from build123d import *

# Parameters (mm, degrees)
HEXBASE_DEPTH             = 2
TUBECLAMPINGHEADS_R       = 5.9
TUBECLAMPINGHEAD_DEPTH    = 2
FASTENINGHEADS_R          = 6.5785
FASTENINGHEAD_DEPTH       = 8
FASTENINGHEAD_TAPER       = 2.5
BOREFASTENINGHEADS_R      = 4.7
BOREFASTENINGHEAD_DEPTH   = 3.2
HEXKEY_DEPTH              = 16.197806859
BORETUBEACCESSS_R         = 5
BORETUBEACCESS_DEPTH      = 9.8
ORINGSEAT_START           = 1.5
ORINGSEATS_R              = 5
ORINGSEATS_R_2            = 4
ORINGSEAT_DEPTH           = 1.5
CHAMFERHEXBASES_OUTSIDE_W = 82.42
CHAMFERHEXBASES_OUTSIDE_H = 80.254
CHAMFERHEXBASES_OUTSIDE_R = 7
CHAMFERHEXBASE_DEPTH      = 17.072751343
CHAMFERHEXBASE_DRAFT      = -60
CHB_VM_COPY_1_SKETCH_W    = 82.42
CHB_VM_COPY_1_SKETCH_H    = 80.254
CHB_VM_COPY_1_SKETCH_R    = 7
CHB_VM_COPY_1_DEPTH       = 17.072751343
CHB_VM_COPY_1_DRAFT       = -60


with BuildPart() as part:
    # HexBaseS → HexBase (new, symmetric)
    with BuildSketch(Plane(origin=(0, 0, 0), x_dir=(1, 0, 0), z_dir=(0, 1, 0))):
        Polygon((8.082903769, 0), (4.041451884, 7), (-4.041451884, 7), (-8.082903769, 0), (-4.041451884, -7), (4.041451884, -7), align=None)
    extrude(amount=HEXBASE_DEPTH, both=True)

    # TubeClampingHeadS → TubeClampingHead (add)
    with BuildSketch(Plane(origin=(0, 2, 0), x_dir=(1, 0, 0), z_dir=(0, 1, 0))):
        with Locations(Location((0, 0, 0), (0, 0, 270))):
            Circle(TUBECLAMPINGHEADS_R)
    extrude(amount=TUBECLAMPINGHEAD_DEPTH)

    # FasteningHeadS → FasteningHead (add)
    with BuildSketch(Plane(origin=(0, -2, 0), x_dir=(-1, 0, 0), z_dir=(0, -1, 0))):
        Circle(FASTENINGHEADS_R)
    extrude(amount=FASTENINGHEAD_DEPTH, taper=FASTENINGHEAD_TAPER)

    # BoreFasteningHeadS → BoreFasteningHead (cut)
    with BuildSketch(Plane.XZ.offset(10)):
        with Locations(Location((0, 0, 0), (0, 0, 270))):
            Circle(BOREFASTENINGHEADS_R)
    extrude(amount=-BOREFASTENINGHEAD_DEPTH, mode=Mode.SUBTRACT)

    # HexKeyS → HexKey (cut, through all)
    with BuildSketch(Plane(origin=(0, -6.8, 0), x_dir=(-1, 0, 0), z_dir=(0, -1, 0))):
        Polygon((-1.443375673, 2.5), (-2.886751346, 0), (-1.443375673, -2.5), (1.443375673, -2.5), (2.886751346, 0), (1.443375673, 2.5), align=None)
    extrude(amount=-HEXKEY_DEPTH, mode=Mode.SUBTRACT)

    # BoreTubeAccessS → BoreTubeAccess (cut)
    with BuildSketch(Plane(origin=(0, 4, 0), x_dir=(1, 0, 0), z_dir=(0, 1, 0))):
        with Locations(Location((0, 0, 0), (0, 0, 270))):
            Circle(BORETUBEACCESSS_R)
    extrude(amount=-BORETUBEACCESS_DEPTH, mode=Mode.SUBTRACT)

    # ClampingFeatureS → ClampingFeature (revolve, cut)
    with BuildSketch(Plane.XY, mode=Mode.PRIVATE) as clampingfeature_sk:
        with BuildLine():
            Line((5, 4), (5.9, 4))
            Line((5.9, 4), (5.9, 3))
            ThreePointArc((5.9, 3), (5.536608024, 3.577947222), (5, 4))
        make_face()
    revolve(clampingfeature_sk.sketch.rotate(Axis((0, 4, 0), (0, -1, 0)), 90), axis=Axis((0, 4, 0), (0, -1, 0)), mode=Mode.SUBTRACT)

    # ORingSeatS → ORingSeat (add)
    with BuildSketch(Plane(origin=(0, -5.8, 0), x_dir=(1, 0, 0), z_dir=(0, 1, 0)).offset(ORINGSEAT_START)):
        with Locations(Location((0, 0, 0), (0, 0, 270))):
            Circle(ORINGSEATS_R)
        with Locations(Location((0, 0, 0), (0, 0, 270))):
            Circle(ORINGSEATS_R_2, mode=Mode.SUBTRACT)
    extrude(amount=-ORINGSEAT_DEPTH)


with BuildPart() as chamferhexbase_tool:
    # ChamferHexBaseS outside → ChamferHexBase (with draft: the straight prism first)
    with BuildSketch(Plane(origin=(0, 2, 0), x_dir=(1, 0, 0), z_dir=(0, 1, 0))):
        Rectangle(CHAMFERHEXBASES_OUTSIDE_W, CHAMFERHEXBASES_OUTSIDE_H)
        Circle(CHAMFERHEXBASES_OUTSIDE_R, mode=Mode.SUBTRACT)
    extrude(amount=-CHAMFERHEXBASE_DEPTH)
    # ChamferHexBase: the draft: its side faces are tilted about the plane it starts from
    chamferhexbase_sides = [chamferhexbase_tool.faces().sort_by_distance(p)[0] for p in [
        (0, -6.536375671, 40.127),
        (41.21, -6.536375671, 0),
        (0, -6.536375671, -40.127),
        (-41.21, -6.536375671, 0),
        (-7, -6.536375671, 0),
    ]]
    draft(chamferhexbase_sides, Plane(origin=(0, 2, 0), x_dir=(1, 0, 0), z_dir=(0, 1, 0)), CHAMFERHEXBASE_DRAFT)


with BuildPart() as part_1:
    add(part.part)

    # ChamferHexBase: cut by chamferhexbase_tool
    add(chamferhexbase_tool.part, mode=Mode.SUBTRACT)


with BuildPart() as chb_vm_copy_1_tool:
    # CHB VM copy 1 sketch → CHB VM copy 1 (with draft: the straight prism first)
    with BuildSketch(Plane.XZ.offset(2)):
        Rectangle(CHB_VM_COPY_1_SKETCH_W, CHB_VM_COPY_1_SKETCH_H)
        Circle(CHB_VM_COPY_1_SKETCH_R, mode=Mode.SUBTRACT)
    extrude(amount=-CHB_VM_COPY_1_DEPTH)
    # CHB VM copy 1: the draft: its side faces are tilted about the plane it starts from
    chb_vm_copy_1_sides = [chb_vm_copy_1_tool.faces().sort_by_distance(p)[0] for p in [
        (0, 6.536375671, 40.127),
        (41.21, 6.536375671, 0),
        (0, 6.536375671, -40.127),
        (-41.21, 6.536375671, 0),
        (-7, 6.536375671, 0),
    ]]
    draft(chb_vm_copy_1_sides, Plane.XZ.offset(2), CHB_VM_COPY_1_DRAFT)


with BuildPart() as part_2:
    add(part_1.part)

    # CHB VM copy 1: cut by chb_vm_copy_1_tool
    add(chb_vm_copy_1_tool.part, mode=Mode.SUBTRACT)


solid = part_2.part
Could you check a few things on this model? Use its own coordinates, in mm. A direction names the side the tool comes from. Coordinates: 2 decimals unless noted, no trailing zeros. Loops run counter-clockwise (first coordinate to the right, second up) from the corner with the lowest first, then second, coordinate; pieces in that order, holes last.
1. We'd pull the mould along Z, two halves only. Please class faces 1 (the face through (-6.034, 0.028, -3.549)), 2 (the face through (6.034, 0.028, 3.549)), 3 (the face through (0, -5.8, 3)): released by +Z, released by -Z, zero draft, split by the parting line, or undercut.
2. For P1, Ø0.5, axis at x = 0.5, y = -6.5, coming from the -Z side; P2, Ø0.8, axis at x = -0.5, y = -6.5, coming from the +Z side; P3, Ø4, axis at x = -3, y = -6.5, coming from the +Z side, each with a flat end and sliding along its axis, tell me the tip position at first contact or that it passes through.
3. For faces 4 (the face through (0, -6, -2.5)), 5 (the face through (1.412, -8.422, -4.483)), 6 (the face through (7.26, -1.85, -0.02)), 7 (the face through (-3.905, -5.04, -0.867)), 8 (the face through (-6.09, 0.03, 3.45)), which set-ups out of +Z, -Z, +X, -X, +Y, -Y let a thin tool reach every point of the face, with its end or its side?
4. I need wall thicknesses on L1, parallel to Y at x = 1.75, z = -4; L2, parallel to Y at x = -2.5, z = 3; L3, parallel to Z at x = 0.5, y = -8. Which ranges of each line are inside material? Lowest first, please.
5. Imagine slicing it at A-A (y = -8.25). Please give me the cut outline in (x, z).
Computed values:
1. face 1: released by -Z
1. face 2: released by +Z
1. face 3: undercut
2. P1: stops at z = -6.38
2. P2: stops at z = 6.39
2. P3: stops at z = 6.31
3. face 4: +Y, -Y
3. face 5: -Y
3. face 6: +X, -Y
3. face 7: +Y
3. face 8: +Z, -X, +Y, -Y
4. L1: y = -6.8 to -4.3
4. L2: y = -6.8 to -5.8
4. L3: z = -6.3 to -4.67, 4.67 to 6.3
5. outline: circle Ø12.61 at (0, 0); hole circle Ø9.4 at (0, 0)
